Geometry check sheet. Reference: the model listing, model coordinates, mm. A direction names the side the tool comes from. Round coordinates to 2 decimals unless told otherwise and drop trailing zeros. Write each loop counter-clockwise with the first axis right and the second up, starting at its lowest first coordinate (ties: lowest second). Pieces come first, ordered by that corner, then holes. Notation, with made-up numbers: (-16.75, -25) -> (21.25, -25) arc R35 ccw to (21.25, 11) -> close; hole circle Ø11 at (82.25, -37.5). An arc over 180 degrees is marked (long way). One line per question, with ' | ' between items.
```python
from build123d import *

# Parameters (mm, degrees)
SKETCH1_W                = 115
SKETCH1_H                = 214
BOSS_EXTRUDE1_DEPTH      = 50
SKETCH4_W                = 25
SKETCH4_H                = 25
CUT_EXTRUDE1_DEPTH       = 249.034271825
SHELL1_START             = 2
SHELL1_OUTLINE_W         = 111
SHELL1_OUTLINE_H         = 185
SHELL1_DEPTH             = 46
SHELL1_2_OUTLINE_W       = 111
SHELL1_2_OUTLINE_H       = 27
SHELL1_2_DEPTH           = 23
M4_CLEARANCE_HOLE1_D     = 4.3
M4_CLEARANCE_HOLE1_DEPTH = 4
M4_CLEARANCE_HOLE1_TIP   = 1.291850331
TAP_DRILL_FOR_M4_TAP1_D  = 3.3


# Read off the part's stored shape, not the designer's step: Shell1
with BuildPart() as part:
    # Sketch1 → Boss-Extrude1 (new body)
    with BuildSketch(Plane(origin=(0, 0, 0), x_dir=(1, 0, 0), z_dir=(0, 1, 0))):
        with Locations((57.5, 107)):
            Rectangle(SKETCH1_W, SKETCH1_H)
    extrude(amount=BOSS_EXTRUDE1_DEPTH)

    # Sketch4 → Cut-Extrude1 (cut, through all)
    with BuildSketch(Plane(origin=(115, 0, 0), x_dir=(0, 0, -1), z_dir=(1, 0, 0))):
        with Locations((201.5, 37.5)):
            Rectangle(SKETCH4_W, SKETCH4_H)
    extrude(amount=-CUT_EXTRUDE1_DEPTH, mode=Mode.SUBTRACT)

    # Shell1 outline → Shell1 (cut)
    with BuildSketch(Plane(origin=(0, 0, 0), x_dir=(1, 0, 0), z_dir=(0, 1, 0)).offset(SHELL1_START)):
        with Locations((57.5, 94.5)):
            Rectangle(SHELL1_OUTLINE_W, SHELL1_OUTLINE_H)
    extrude(amount=SHELL1_DEPTH, mode=Mode.SUBTRACT)

    # Shell1 2 outline → Shell1 2 (cut)
    with BuildSketch(Plane(origin=(0, 0, 0), x_dir=(1, 0, 0), z_dir=(0, 1, 0)).offset(SHELL1_START)):
        with Locations((57.5, 200.5)):
            Rectangle(SHELL1_2_OUTLINE_W, SHELL1_2_OUTLINE_H)
    extrude(amount=SHELL1_2_DEPTH, mode=Mode.SUBTRACT)

    # M4 Clearance Hole1
    with Locations(Plane(origin=(0, 0, 0), x_dir=(-1, 0, 0), z_dir=(0, -1, 0))):
        with Locations((-32.5, 32), (-57.5, 107), (-32.5, 182), (-82.5, 32), (-82.5, 182)):
            Hole(M4_CLEARANCE_HOLE1_D / 2, depth=M4_CLEARANCE_HOLE1_DEPTH)
            with Locations((0, 0, -(M4_CLEARANCE_HOLE1_DEPTH + M4_CLEARANCE_HOLE1_TIP / 2))):  # 118° drill point
                Cone(0, M4_CLEARANCE_HOLE1_D / 2, M4_CLEARANCE_HOLE1_TIP, mode=Mode.SUBTRACT)

    # Tap Drill for M4 Tap1 (through all)
    with Locations(Plane(origin=(115, 0, 0), x_dir=(0, 0, -1), z_dir=(1, 0, 0))):
        with Locations((181.5, 33)):
            Hole(TAP_DRILL_FOR_M4_TAP1_D / 2)


solid = part.part
```
(1) Draft check along Y on faces 1 (the flat face through (113, 25, -107)), 2 (the cylindrical face through (82.03, 1.01, -179.9)), 3 (the flat face through (44, 0, -108)), 4 (the flat face through (57, 25, -2)). Enter one of: +Y half, -Y half, draft (parallel to the pull), parting line (faces both ways), or undercut.
Resolved:
face 1: undercut | face 2: draft | face 3: -Y half | face 4: undercut
(2) Material ranges on line 1 (Z direction, x = 82.5, y = 1.55); line 2 (X direction, y = 1.1, z = -32); line 3 (Y direction, x = 76, z = -12.5), recorded low to high.
Resolved:
line 1: z = -214 to -184.15, -179.85 to -34.15, -29.85 to 0 | line 2: x = 0 to 30.35, 34.65 to 80.35, 84.65 to 115 | line 3: y = 0 to 2, 48 to 50
(3) Sectioned sample at B-B on x = 32.5. Record the cut outline in (y, z).
Resolved:
outline: (0, -214) -> (2, -214) -> (2, -184.15) -> (0, -184.15) -> close; (0, -179.85) -> (2, -179.85) -> (2, -34.15) -> (0, -34.15) -> close; (0, -29.85) -> (2, -29.85) -> (2, -2) -> (48, -2) -> (48, -187) -> (25, -187) -> (25, -189) -> (50, -189) -> (50, 0) -> (0, 0) -> close
(4) Sectioned sample at C-C on y = 5.5. Record the cut outline in (x, z), then the cut area to 3 significant figures.
Resolved:
outline: (0, -214) -> (2, -214) -> (2, -2) -> (113, -2) -> (113, -214) -> (115, -214) -> (115, 0) -> (0, 0) -> close | area: 1,080 mm2
(5) Go/stop test with flat-tipped pins: pin 1 (3.5 mm diameter, centred on x = 32.5, z = -32, fed in from -Y); pin 2 (2 mm diameter, centred on y = 33, z = -181.5, fed in from -X); pin 3 (3 mm diameter, centred on y = 7.5, z = -132.5, fed in from -X); pin 4 (5 mm diameter, centred on x = 80, y = 21, fed in from -Z). Record where each tip stops, or that it passes through.
Resolved:
pin 1: stops at y = 48 | pin 2: passes through | pin 3: stops at x = 0 | pin 4: stops at z = -2
(6) Sectioned sample at D-D on x = 69.5. Record the cut outline in (y, z).
Resolved:
outline: (0, -214) -> (2, -214) -> (2, -2) -> (48, -2) -> (48, -187) -> (25, -187) -> (25, -189) -> (50, -189) -> (50, 0) -> (0, 0) -> close
(7) Sectioned sample at A-A on z = -32. Record the cut outline in (x, y).
Resolved:
outline: (0, 0) -> (30.35, 0) -> (30.35, 2) -> (2, 2) -> (2, 48) -> (113, 48) -> (113, 2) -> (84.65, 2) -> (84.65, 0) -> (115, 0) -> (115, 50) -> (0, 50) -> close; (34.65, 0) -> (80.35, 0) -> (80.35, 2) -> (34.65, 2) -> close
(8) Access from +Z, -Z, +X, -X, +Y, -Y to the whole of each face (thin tool, end or side, straight path). Record for faces 5 (the flat face through (57, 48, -96)), 6 (the cylindrical face through (32.03, 1.01, -179.9)), 7 (the flat face through (40, 1, -214)), 8 (the flat face through (58, 37, -189)), 9 (the flat face through (56.7, 2, -109.5)).
Resolved:
face 5: none | face 6: -Y | face 7: -Z, +X, -X, +Y, -Y | face 8: -Z, +X, -X, +Y | face 9: -Z
